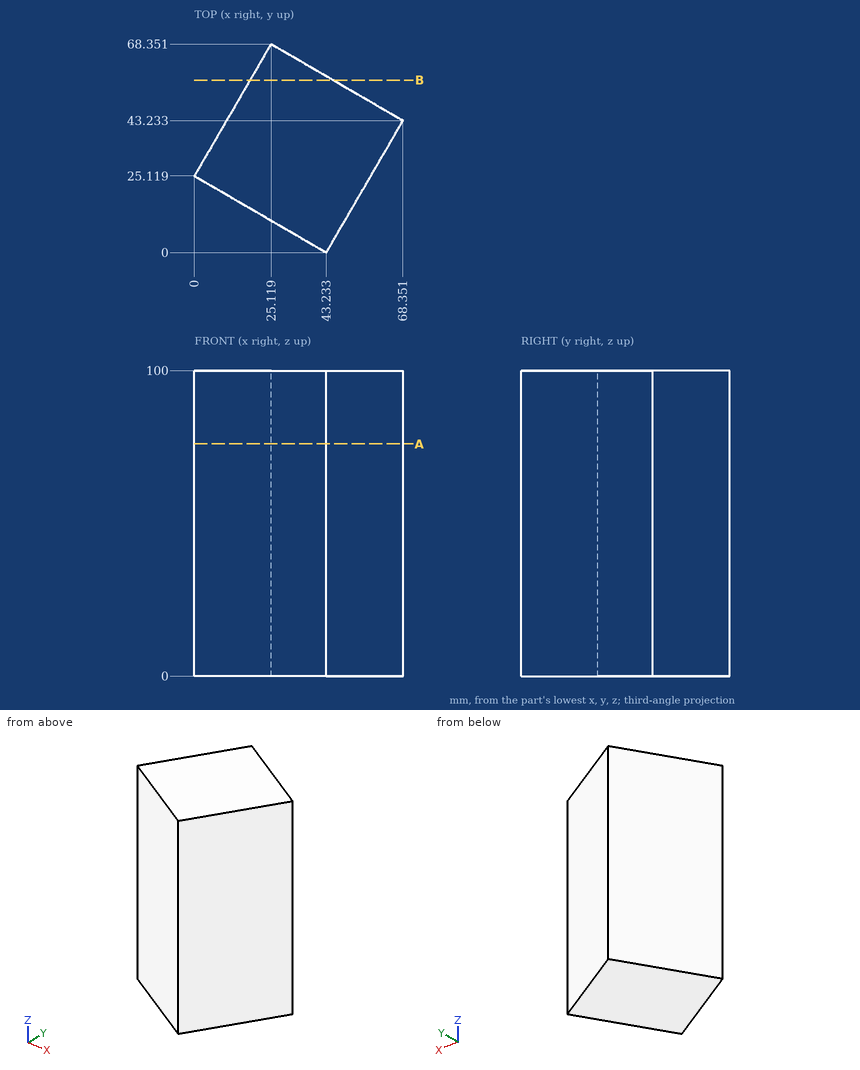
Verification items for this drawing (mm, ordinates from the low corner). Coordinates: 2 decimals unless noted, no trailing zeros. Order: outer loops, then holes, each group sorted by start corner. A loop starts at its lowest first (then second) coordinate and runs counter-clockwise, first axis right, second up. Notation, with made-up numbers: (86.5, 30.25) -> (100.5, 30.25) arc R14 cw to (100.5, 44.25) -> close; hole circle Ø4 at (31, -40). An arc over 180 degrees is marked (long way). Answer as CSV lines item,"result". Start each with the question number.
1) Gauge pin test, flat ends, axial feed: pin 1 Ø3 at (y, z) = (36, 55) entering from +X; pin 2 Ø1.5 at (x, z) = (35.5, 17) entering from +Y (1 decimal); pin 3 Ø2 at (y, z) = (49.5, 54) entering from -X (1 decimal); pin 4 Ø8 at (x, y) = (19.5, 53) entering from -Z. Record the tip position at first contact, or that the pin passes through.
2) Cross-section at B-B, the plane y = 56.5. Record the boundary of the cut face in (x, z), then the cut area to 3 significant figures.
3) Material ranges on L1, parallel to Y at x = 19, z = 28.5; L2, parallel to X at y = 28.5, z = 22 (1 decimal); L3, parallel to X at y = 40.5, z = 44.5 (1 decimal), recorded low to high. Write a range as [from, to].
4) Cross-section at A-A, the plane z = 76. Record the boundary of the cut face in (x, y).
Conclusion:
1,pin 1,"stops at x = 65.02"
1,pin 2,"stops at y = 62.8"
1,pin 3,"stops at x = 13.6"
1,pin 4,"stops at z = 0"
2,outline,"(18.23, 0) -> (45.52, 0) -> (45.52, 100) -> (18.23, 100) -> close"
2,area,"2,730 mm²"
3,L1,"y = [14.08, 57.82]"
3,L2,"x = [2, 59.8]"
3,L3,"x = [8.9, 66.8]"
4,outline,"(0, 25.12) -> (43.23, 0) -> (68.35, 43.23) -> (25.12, 68.35) -> close"
